Autodesk Inventor part; units mm, degrees
ref_plane "YZ Plane" through (0, 0, 0) normal (1, 0, 0) x (0, 1, 0)
ref_plane "XZ Plane" through (0, 0, 0) normal (0, 1, 0) x (-1, 0, 0)
ref_plane "XY Plane" through (0, 0, 0) normal (0, 0, 1) x (1, 0, 0)
sketch "Sketch1" plane through (0, 0, 0) normal (0, 0, 1) x (1, 0, 0)
  line L0 (-265.2211, 0) -> (0, 0)
  line L1 (0, 0) -> (0, -436.8243)
  arc A0 (-200, 0) -> (0, -200) centre (0, 0) ccw
  line L2 (-200, 0) -> (-200, 50)
  line L3 (0, -200) -> (50, -200)
  dimension "d30" = 400
  dimension "d31" = 50
  dimension "d32" = 50
ref_plane "Work Plane1" through (-200, 50, 0) normal (0, 1, 0) x (-1, 0, 0)
sketch "Sketch2" plane through (-200, 50, 0) normal (0, 1, 0) x (-1, 0, 0)
  circle A0 centre (0, 0) radius 75
  circle A1 centre (0, 0) radius 37.5
  circle A2 centre (62.5, 0) radius 5
  circle A3 centre (31.25, 54.1266) radius 5
  circle A4 centre (-31.25, 54.1266) radius 5
  circle A5 centre (-62.5, 0) radius 5
  circle A6 centre (-31.25, -54.1266) radius 5
  circle A7 centre (31.25, -54.1266) radius 5
  point P0 (-200, 0)
  dimension "d3" = 150
  dimension "d4" = 75
  dimension "d5" = 10
  dimension "d6" = 62.5
  dimension "d9" = 360
sketch "Sketch3" plane through (-200, 50, 0) normal (0, 1, 0) x (-1, 0, 0)
  circle A0 centre (0, 0) radius 50
  circle A1 centre (0, 0) radius 37.5
  point P0 (-200, 0)
  dimension "d11" = 100
  dimension "d12" = 75
sweep "Sweep2" add profiles "Sketch3" path "Sketch1" path curves L2 A0 L3
extrude "Extrusion3" add sketch "Sketch2" along normal blind 20
sketch "Sketch5" plane through (50, -200, 0) normal (1, 0, 0) x (0, 0, -1)
  circle A0 centre (0, 0) radius 75
  circle A1 centre (0, 0) radius 37.5
  circle A2 centre (62.5, 0) radius 5
  circle A3 centre (31.25, 54.1266) radius 5
  circle A4 centre (-31.25, 54.1266) radius 5
  circle A5 centre (-62.5, 0) radius 5
  circle A6 centre (-31.25, -54.1266) radius 5
  circle A7 centre (31.25, -54.1266) radius 5
  point P0 (0, 200)
  dimension "d39" = 150
  dimension "d40" = 75
  dimension "d41" = 10
  dimension "d42" = 62.5
  dimension "d43" = 360
extrude "Extrusion4" add sketch "Sketch5" along normal blind 20
equation "\"d30\" = Elbow_Diameter"
equation "\"d31\" = Elbow_Length"
equation "\"d32\" = Elbow_Length"
equation "\"d3\" = Flange_Diameter"
equation "\"d4\" = Inner_Diameter"
equation "\"d5\" = Hole_Diameter"
equation "\"d6\" = Hole_Position"
equation "\"d11\" = Outer_Diameter"
equation "\"d12\" = Inner_Diameter"
equation "\"d35\" = Flange_Hight"
equation "\"d39\" = Flange_Diameter"
equation "\"d40\" = Inner_Diameter"
equation "\"d41\" = Hole_Diameter"
equation "\"d42\" = Hole_Position"
equation "\"d48\" = Flange_Hight"
equation "\"Elbow_Diameter\" = 400"
equation "\"Elbow_Length\" = 50"
equation "\"Flange_Diameter\" = 150"
equation "\"Inner_Diameter\" = 75"
equation "\"Fillet_Radius\" = 6"
equation "\"Flange_Hight\" = 20"
equation "\"Hole_Position\" = 0.166667 * Inner_Diameter + 0.333333 * Flange_Diameter"
equation "\"Hole_Diameter\" = 10"
equation "\"Outer_Diameter\" = 100"
properties part number "Parametric" material "Steel, Mild"
Model file for the job. Use its own axes, mm. A direction names the side the tool comes from. Give positions to 0.01 mm unless a question says otherwise; leave off trailing zeros. Write each loop counter-clockwise with the first axis right and the second up, starting at its lowest first coordinate (ties: lowest second). Pieces come first, ordered by that corner, then holes. Notation, with made-up numbers: (-10.75, 61) -> (9.25, 61) arc R31 cw to (9.25, 92) -> close; hole circle Ø6 at (51, -13.75). An arc over 180 degrees is marked (long way). Write item = value, one per line.
(1) Probe line 1 along X through (y, z) = (32, 0); line 2 along Z through (x, y) = (-231.25, 57.5); line 3 along X through (y, z) = (-245, 22.5). List the from-to ranges inside material, lowest first.
Determined:
line_1 = -250 to -237.5, -162.5 to -150
line_2 = -68.18 to -59.13, -49.13 to -20.73, 20.73 to 49.13, 59.13 to 68.18
line_3 = 50 to 70
(2) Slice it at B-B, the plane y = -200. Give the number of separate pieces and of enclosed holes in the cut face, then the cut area to 3 significant figures.
Determined:
separate_pieces = 3
enclosed_holes = 0
area = 7,000 mm2
(3) Tool access for faces 4 (the face through (-235.87, 59.86, -52.21)), 5 (the face through (-142.27, 59.86, -1.5)), 6 (the face through (59.86, -274.362, 9.764)), 7 (the face through (24.65, -150.05, 2.2)): list every direction of +Z, -Z, +X, -X, +Y, -Y with a clear straight run to the whole face (end or side of a thin tool).
Determined:
face_4 = +Y, -Y
face_5 = +Y
face_6 = +X
face_7 = none
(4) Slice it at A-A, the plane x = -262.5. Give the cut face in (y, z).
Determined:
outline = (50, -41.46) -> (70, -41.46) -> (70, -5) -> (50, -5) -> close; (50, 5) -> (70, 5) -> (70, 41.46) -> (50, 41.46) -> close
(5) Flat gauge pins, fed straight in: P1, Ø4, axis at y = -121, z = -1.5, coming from the -X side; P2, Ø13, axis at y = -254.13, z = 31.25, coming from the +X side; P3, Ø6, axis at y = -254.13, z = -31.25, coming from the -X side; P4, Ø12, axis at x = -155, y = -114.5, coming from the -Z side. Where does each tip first touch, or does it go through?
Determined:
P1 = -219.84
P2 = 70
P3 = through
P4 = -49.98
(6) Slice it at D-D, the plane x = 9.5. Give the cut face in (y, z).
Determined:
outline = circle Ø100 at (-200, 0); hole circle Ø75 at (-200, 0)
(7) Mould opens along Y. For faces 1 (the face through (59.86, -257.506, 34.935)), 2 (the face through (-164.782, 59.86, 57.169)), 3 (the face through (-165.6, 70, -15.6)) say: released by +Y, released by -Y, zero draft, split by the parting line, or undercut.
Determined:
face_1 = undercut
face_2 = zero draft
face_3 = released by +Y
